Geometry: final body of the model. Coordinates: model frame, mm. A direction names the side the tool comes from. Give positions to 0.01 mm unless a question says otherwise; leave off trailing zeros. Write each loop counter-clockwise with the first axis right and the second up, starting at its lowest first coordinate (ties: lowest second). Pieces come first, ordered by that corner, then holes. Notation, with made-up numbers: (15, -39.5) -> (42, -39.5) arc R14 cw to (42, -20.5) -> close; hole circle Ø6 at (31.5, 49). An arc over 180 degrees is marked (long way). Answer in a Markdown table with one row per item. Add a question column.
Item 1: Section query B-B on y = 28. Output: boundary loops of the cut face in (x, z) (3 decimals), plus the area to 3 significant figures.
Item 2: Section query A-A on z = 6. Output: boundary loops of the cut face in (x, y).
Item 3: Material intervals for probe 1 along Z at (x, y) = (80, 60) (3 decimals); probe 2 along Z at (x, y) = (81.75, 4); probe 3 along Y at (x, z) = (80.75, 16.5), sorted ascending. Write a range as from..to.
Item 4: Draft query along Y for faces 5 (the flat face through (79, 48, 0)), 6 (the flat face through (79, 6.35, 6)), 7 (the flat face through (79, 0, 38)), 8 (the flat face through (79, 101.6, 67)). Return one class per face: +Y half, -Y half, draft (parallel to the pull), parting line (faces both ways), or undercut.
Item 5: Section query C-C on x = 78.5. Output: boundary loops of the cut face in (y, z) (3 decimals), plus the area to 3 significant figures.
Item 6: First-contact query: P1, Ø1.9, axis at x = 78.5, y = 98.5, coming from the +Z side. Flat tip, straight axial feed; report the tip coordinate or a pass-through.
Item 7: Section query D-D on z = 39.5. Output: boundary loops of the cut face in (x, y).
Item 8: Access query for faces 1 (the flat face through (79, 47, 3.175)), 2 (the flat face through (79, 95.25, 38)), 3 (the flat face through (79, 95, 69.85)), 4 (the flat face through (79, 0, 69.85)). Directions: +Z, -Z, +X, -X, +Y, -Y. A direction counts if a zero-diameter tool reaches every point of the face in a straight line with its end or side. Return the directions, or none.
```python
from build123d import *

# Parameters (mm, degrees)
SKETCH1_W           = 6.35
SKETCH1_H           = 107.95
BOSS_EXTRUDE1_DEPTH = 76.2
SKETCH2_W           = 6.35
SKETCH2_H           = 12.7
SKETCH2_W_2         = 50.8
SKETCH2_H_2         = 6.35
SKETCH2_H_3         = 82.55
CUT_EXTRUDE1_DEPTH  = 128.158650905


with BuildPart() as part:
    # Sketch1 → Boss-Extrude1 (new body)
    with BuildSketch(Plane.XY):
        with Locations((79.375, 47.625)):
            Rectangle(SKETCH1_W, SKETCH1_H)
    extrude(amount=BOSS_EXTRUDE1_DEPTH)

    # Sketch2 → Cut-Extrude1 (cut, through all)
    with BuildSketch(Plane(origin=(82.55, 0, 0), x_dir=(0, 0, -1), z_dir=(1, 0, 0))):
        with Locations((-73.025, 95.25)):
            Rectangle(SKETCH2_W, SKETCH2_H)
        with Locations((-73.025, 0)):
            Rectangle(SKETCH2_W, SKETCH2_H)
        with Locations((-38.1, 98.425)):
            Rectangle(SKETCH2_W_2, SKETCH2_H_2)
        with Locations((-6.35, 47.625)):
            Rectangle(SKETCH2_W, SKETCH2_H_3)
        with Locations((-38.1, -3.175)):
            Rectangle(SKETCH2_W_2, SKETCH2_H_2)
    extrude(amount=-CUT_EXTRUDE1_DEPTH, mode=Mode.SUBTRACT)


solid = part.part
```
Findings below:
| question | item | result |
|---|---|---|
| 1 | outline | (76.2, 0) -> (82.55, 0) -> (82.55, 3.175) -> (76.2, 3.175) -> close; (76.2, 9.525) -> (82.55, 9.525) -> (82.55, 76.2) -> (76.2, 76.2) -> close |
| 1 | area | 444 mm^2 |
| 2 | outline | (76.2, -6.35) -> (82.55, -6.35) -> (82.55, 6.35) -> (76.2, 6.35) -> close; (76.2, 88.9) -> (82.55, 88.9) -> (82.55, 101.6) -> (76.2, 101.6) -> close |
| 3 | probe 1 | z = 0..3.175, 9.525..76.2 |
| 3 | probe 2 | z = 0..69.85 |
| 3 | probe 3 | y = 0..95.25 |
| 4 | face 5 | draft |
| 4 | face 6 | undercut |
| 4 | face 7 | -Y half |
| 4 | face 8 | +Y half |
| 5 | outline | (-6.35, 0) -> (101.6, 0) -> (101.6, 12.7) -> (95.25, 12.7) -> (95.25, 63.5) -> (101.6, 63.5) -> (101.6, 69.85) -> (88.9, 69.85) -> (88.9, 76.2) -> (6.35, 76.2) -> (6.35, 69.85) -> (-6.35, 69.85) -> (-6.35, 63.5) -> (0, 63.5) -> (0, 12.7) -> (-6.35, 12.7) -> close; hole (6.35, 3.175) -> (88.9, 3.175) -> (88.9, 9.525) -> (6.35, 9.525) -> close |
| 5 | area | 6,900 mm^2 |
| 6 | P1 | stops at z = 69.85 |
| 7 | outline | (76.2, 0) -> (82.55, 0) -> (82.55, 95.25) -> (76.2, 95.25) -> close |
| 8 | face 1 | +X, -X |
| 8 | face 2 | +X, -X, +Y |
| 8 | face 3 | +Z, +X, -X, +Y |
| 8 | face 4 | +Z, +X, -X, -Y |
